Can you work these out from the drawing? Everything is in mm from the part's minimum corner. A direction names the side the tool comes from. Give positions to 0.01 mm unless a question says otherwise; leave off trailing zeros. Loops run counter-clockwise (first coordinate to the right, second up) from the corner with the lowest first, then second, coordinate; pieces in that order, holes last. Notation, with made-up numbers: (73.5, 30) - (89.5, 30) arc R11 ccw to (89.5, 50) - close; hole circle Ø8 at (22.5, 12.25). An arc over 180 degrees is marked (long way). Answer in a Markdown table with one row per item.
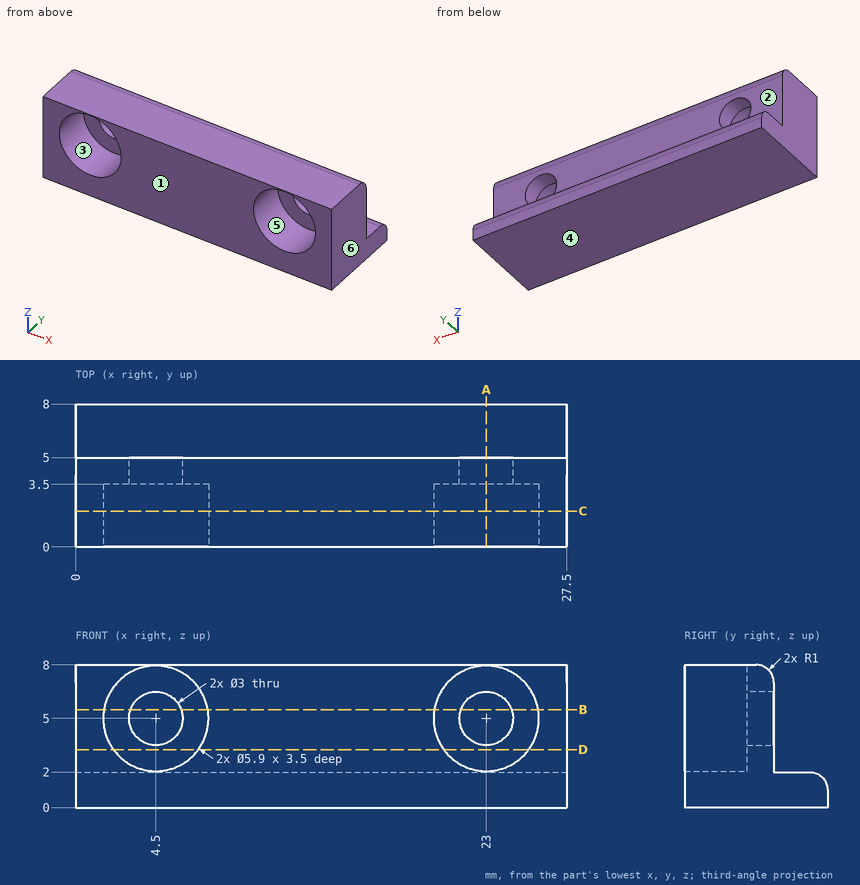
Q1. Imagine slicing it at B-B, the plane z = 5.5. Write out the boundary of the cut face in (x, y), and give its area (3 significant figures).
Checked values:
| item | result |
|---|---|
| outline | (0, 0) - (1.59, 0) - (1.59, 3.5) - (3.09, 3.5) - (3.09, 5) - (0, 5) - close; (5.91, 3.5) - (7.41, 3.5) - (7.41, 0) - (20.09, 0) - (20.09, 3.5) - (21.59, 3.5) - (21.59, 5) - (5.91, 5) - close; (24.41, 3.5) - (25.91, 3.5) - (25.91, 0) - (27.5, 0) - (27.5, 5) - (24.41, 5) - close |
| area | 88.3 mm² |
Q2. Imagine slicing it at A-A, the plane x = 23. Write out the boundary of the cut face in (y, z).
Checked values:
| item | result |
|---|---|
| outline | (0, 0) - (8, 0) - (8, 1) arc R1 ccw to (7, 2) - (5, 2) - (5, 3.5) - (3.5, 3.5) - (3.5, 2.05) - (0, 2.05) - close; (0, 7.95) - (3.5, 7.95) - (3.5, 6.5) - (5, 6.5) - (5, 7) arc R1 ccw to (4, 8) - (0, 8) - close |
Q3. On a 3-axis mill with a long thin cutter (end or side, diameter ignored), from which of +Z, -Z, +X, -X, +Y, -Y can I reach the whole of each face in a straight line? I mean the marked faces 1 and 2. Say none if no direction works.
Checked values:
| item | result |
|---|---|
| face 1 | +Z, -Z, +X, -X, -Y |
| face 2 | +Z, +X, -X, +Y |
Q4. For pin 1 (3.5 mm diameter, centred on x = 4.5, z = 5, fed in from +Y); pin 2 (0.6 mm diameter, centred on x = 10, y = 5.5, fed in from +Z), each with a flat end and sliding along its axis, tell me the tip position at first contact or that it passes through.
Checked values:
| item | result |
|---|---|
| pin 1 | stops at y = 5 |
| pin 2 | stops at z = 2 |
Q5. Imagine slicing it at C-C, the plane y = 2. Write out the boundary of the cut face in (x, z), and give its area (3 significant figures).
Checked values:
| item | result |
|---|---|
| outline | (0, 0) - (27.5, 0) - (27.5, 8) - (0, 8) - close; hole circle Ø5.9 at (4.5, 5); hole circle Ø5.9 at (23, 5) |
| area | 165 mm² |
Q6. Imagine slicing it at D-D, the plane z = 3.25. Write out the boundary of the cut face in (x, y).
Checked values:
| item | result |
|---|---|
| outline | (0, 0) - (2.13, 0) - (2.13, 3.5) - (6.87, 3.5) - (6.87, 0) - (20.63, 0) - (20.63, 3.5) - (25.37, 3.5) - (25.37, 0) - (27.5, 0) - (27.5, 5) - (0, 5) - close |
Q7. If I drill on line 1 (X direction, y = 4.15, z = 5); line 2 (Y direction, x = 7.5, z = 3.5); line 3 (Z direction, x = 13.25, y = 5.5), over which ranges is the centre line in solid material (lowest first)? Write a range as [from, to].
Checked values:
| item | result |
|---|---|
| line 1 | x = [0, 3], [6, 21.5], [24.5, 27.5] |
| line 2 | y = [0, 5] |
| line 3 | z = [0, 2] |
Q8. If we mould it in two halves opening along Z, with no side actions, what happens to the marked faces 3, 4, 5 and 6? For each: released by +Z, released by -Z, zero draft, split by the parting line, or undercut.
Checked values:
| item | result |
|---|---|
| face 3 | undercut |
| face 4 | released by -Z |
| face 5 | undercut |
| face 6 | zero draft |
